```python
from build123d import *

# Parameters (mm, degrees)
BOSS_EXTRUDE1_DEPTH = 6.35
SKETCH2_R           = 0.72
BOSS_EXTRUDE2_DEPTH = 0.48
SKETCH3_R           = 0.72
BOSS_EXTRUDE3_DEPTH = 0.48
SKETCH4_R           = 0.72
BOSS_EXTRUDE4_DEPTH = 0.48
SKETCH5_R           = 0.7
BOSS_EXTRUDE5_DEPTH = 0.48
SKETCH6_R           = 0.7
BOSS_EXTRUDE6_DEPTH = 0.48
SKETCH7_R           = 0.7
BOSS_EXTRUDE7_DEPTH = 0.48
SKETCH8_R           = 0.7
BOSS_EXTRUDE8_DEPTH = 0.48
CUT_EXTRUDE1_DEPTH  = 7.35


with BuildPart() as part:
    # Sketch1 → Boss-Extrude1 (new body)
    with BuildSketch(Plane.XY):
        Polygon((-7.764898793, 19.101651031), (-18.997519567, 8.016294384), (-19.101651031, -7.764898793), (-8.016294384, -18.997519567), (7.764898793, -19.101651031), (18.997519567, -8.016294384), (19.101651031, 7.764898793), (8.016294384, 18.997519567), align=None)
    extrude(amount=BOSS_EXTRUDE1_DEPTH)

    # Sketch2 → Boss-Extrude2 (add)
    with BuildSketch(Plane(origin=(0.125697795, 19.049585299, 0), x_dir=(0.999978231, -0.006598309, 0), z_dir=(0.006598309, 0.999978231, 0))):
        with Locations((-6.239768363, -3.175)):
            Circle(SKETCH2_R)
    extrude(amount=BOSS_EXTRUDE2_DEPTH)

    # Sketch3 → Boss-Extrude3 (add)
    with BuildSketch(Plane(origin=(-13.38120918, 13.558972707, 0), x_dir=(0.711757097, 0.702425679, 0), z_dir=(-0.702425679, 0.711757097, 0))):
        with Locations((-6.239768363, -3.175)):
            Circle(SKETCH3_R)
        with Locations((-0.039768363, -3.175)):
            Circle(SKETCH3_R)
    extrude(amount=BOSS_EXTRUDE3_DEPTH)

    # Sketch4 → Boss-Extrude4 (add)
    with BuildSketch(Plane(origin=(-19.049585299, 0.125697795, 0), x_dir=(0, 0, 1), z_dir=(-0.999978231, 0.006598309, 0))):
        with Locations((3.175, -6.239768363)):
            Circle(SKETCH4_R)
        with Locations((3.175, 0.000224237)):
            Circle(SKETCH4_R)
        with Locations((3.175, 6.240224237)):
            Circle(SKETCH4_R)
    extrude(amount=BOSS_EXTRUDE4_DEPTH)

    # Sketch5 → Boss-Extrude5 (add)
    with BuildSketch(Plane(origin=(-13.558972707, -13.38120918, 0), x_dir=(0, 0, 1), z_dir=(-0.711757097, -0.702425679, 0))):
        with Locations((3.175, -6.239768363)):
            Circle(SKETCH5_R)
        with Locations((3.175, 6.160231637)):
            Circle(SKETCH5_R)
    extrude(amount=BOSS_EXTRUDE5_DEPTH)

    # Sketch6 → Boss-Extrude6 (add)
    with BuildSketch(Plane(origin=(-0.125697795, -19.049585299, 0), x_dir=(-0.999978231, 0.006598309, 0), z_dir=(-0.006598309, -0.999978231, 0))):
        with Locations((-0.039768363, -3.175)):
            Circle(SKETCH6_R)
        with Locations((6.160231637, -3.175)):
            Circle(SKETCH6_R)
    extrude(amount=BOSS_EXTRUDE6_DEPTH)

    # Sketch7 → Boss-Extrude7 (add)
    with BuildSketch(Plane(origin=(13.38120918, -13.558972707, 0), x_dir=(-0.711757097, -0.702425679, 0), z_dir=(0.702425679, -0.711757097, 0))):
        with Locations((-0.039768363, -3.175)):
            Circle(SKETCH7_R)
    extrude(amount=BOSS_EXTRUDE7_DEPTH)

    # Sketch8 → Boss-Extrude8 (add)
    with BuildSketch(Plane(origin=(19.049585299, -0.125697795, 0), x_dir=(0, 0, -1), z_dir=(0.999978231, -0.006598309, 0))):
        with Locations((-3.175, -6.160231637)):
            Circle(SKETCH8_R)
    extrude(amount=BOSS_EXTRUDE8_DEPTH)

    # Sketch9 → Cut-Extrude1 (cut, through all)
    with BuildSketch(Plane(origin=(0, 0, 0), x_dir=(-1, 0, 0), z_dir=(0, 0, -1))):
        Polygon((-3.872311644, 6.226438458), (-7.328409701, -0.240301026), (-3.456098057, -6.466739484), (3.872311644, -6.226438458), (7.328409701, 0.240301026), (3.456098057, 6.466739484), align=None)
    extrude(amount=-CUT_EXTRUDE1_DEPTH, mode=Mode.SUBTRACT)


solid = part.part
```
Geometry: final body of the model. Coordinates: model frame, mm. Round coordinates to 2 decimals unless told otherwise and drop trailing zeros. Order: outer loops, then holes, each group sorted by start corner. A loop starts at its lowest first (then second) coordinate and runs counter-clockwise, first axis right, second up. Notation, with made-up numbers: (60, 22.5) -> (98, 22.5) arc R25 cw to (98, 38.5) -> close; hole circle Ø7 at (46.5, 7). An arc over 180 degrees is marked (long way). Use CSV: the item, a comma, the result in double quotes. Start each with the question number.
1) Section A-A (z = 5.5). Return the cut outline in (x, y), and give its area (3 significant figures).
2) Material intervals for line 1 along X through (y, z) = (-2, 0.5); line 2 along X through (y, z) = (4, 1.5); line 3 along X through (y, z) = (7.5, 5), sorted ascending. Write a range as from..to.
3) Section C-C (x = 2). Return the cut outline in (y, z).
4) First-contact query: pin 1 Ø1 at (x, z) = (10, 1.5) entering from +Y; pin 2 Ø1 at (y, z) = (15, 1) entering from +X; pin 3 Ø1 at (y, z) = (9, 4) entering from +X. Flat tips, straight axial feed; report the tip coordinate or a pass-through.
5) Draft query along X for faces 1 (the face through (13.75, -13.87, 3.17)), 2 (the face through (-17.618, -9.605, 3.498)), 3 (the face through (-13.75, 13.87, 3.16)). Return one class per face: +X half, -X half, draft (parallel to the pull), parting line (faces both ways), or undercut.
6) Section D-D (y = 10.5). Return the cut outline in (x, z), and give its area (3 significant figures).
7) Section B-B (y = 4.5). Return the cut outline in (x, z) (3 decimals), and give its area (3 significant figures).
Returned:
1,outline,"(-19.1, -7.76) -> (-8.02, -19) -> (7.76, -19.1) -> (19, -8.02) -> (19.1, 7.76) -> (8.02, 19) -> (-7.76, 19.1) -> (-19, 8.02) -> close; hole (-7.33, 0.24) -> (-3.87, -6.23) -> (3.46, -6.47) -> (7.33, -0.24) -> (3.87, 6.23) -> (-3.46, 6.47) -> close"
1,area,"1,060 mm²"
2,line 1,"x = -19.06..-6.13, 6.23..19.04"
2,line 2,"x = -19.02..-4.99, 5.06..19.08"
2,line 3,"x = -19..19.1"
3,outline,"(-19.06, 0) -> (-6.42, 0) -> (-6.42, 6.35) -> (-19.06, 6.35) -> close; (6.29, 0) -> (19.04, 0) -> (19.04, 6.35) -> (6.29, 6.35) -> close"
4,pin 1,"stops at y = 17.49"
4,pin 2,"stops at x = 12.45"
4,pin 3,"stops at x = 18.38"
5,face 1,"+X half"
5,face 2,"undercut"
5,face 3,"-X half"
6,outline,"(-16.48, 0) -> (16.4, 0) -> (16.4, 6.35) -> (-16.48, 6.35) -> close"
6,area,"209 mm²"
7,outline,"(-19.021, 0) -> (-4.679, 0) -> (-4.679, 6.35) -> (-19.021, 6.35) -> close; (4.795, 0) -> (19.08, 0) -> (19.08, 6.35) -> (4.795, 6.35) -> close"
7,area,"182 mm²"
